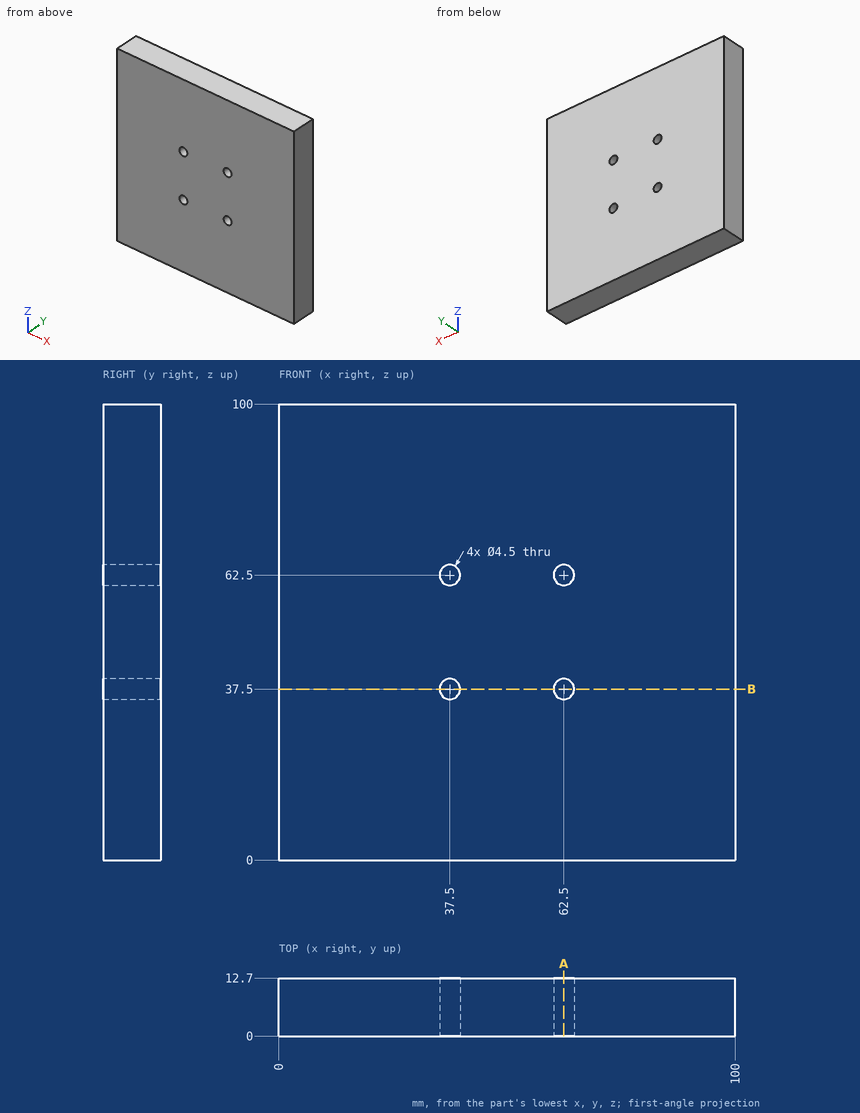
The drawing under review shows one solid part. Ordinate dimensions are in mm from its lowest x, y, z. Round coordinates to 2 decimals unless told otherwise and drop trailing zeros. Write each loop counter-clockwise with the first axis right and the second up, starting at its lowest first coordinate (ties: lowest second). Pieces come first, ordered by that corner, then holes. Notation, with made-up numbers: M 39,-19.5 L 88,-19.5 A37 cw 88,17.5 Z; hole C 27,-24.5 d9. An arc over 180 degrees is marked long. One line per item, written item: value. Start each with the question number.
(1) Wall thickness on line 1 (X direction, y = 3, z = 62.5); line 2 (Z direction, x = 39, y = 9.25); line 3 (Z direction, x = 62, y = 9.25): over which ranges is each line inside the solid? List them lowest first.
(2) We need section A-A (x = 62.5). Give the boundary of the cut face in (y, z).
(3) We need section B-B (z = 37.5). Give the boundary of the cut face in (x, y).
Result:
1. line 1: 0 to 35.25, 39.75 to 60.25, 64.75 to 100
1. line 2: 0 to 35.82, 39.18 to 60.82, 64.18 to 100
1. line 3: 0 to 35.31, 39.69 to 60.31, 64.69 to 100
2. outline: M 0,0 L 12.7,0 L 12.7,35.25 L 0,35.25 Z; M 0,39.75 L 12.7,39.75 L 12.7,60.25 L 0,60.25 Z; M 0,64.75 L 12.7,64.75 L 12.7,100 L 0,100 Z
3. outline: M 0,0 L 35.25,0 L 35.25,12.7 L 0,12.7 Z; M 39.75,0 L 60.25,0 L 60.25,12.7 L 39.75,12.7 Z; M 64.75,0 L 100,0 L 100,12.7 L 64.75,12.7 Z
